Source: CAD feature listing. Evaluate the final solid. Frame: model axes, mm. A direction names the side the tool comes from. Give positions to 0.01 mm unless a question says otherwise; leave off trailing zeros. Loops run counter-clockwise (first coordinate to the right, second up) from the corner with the lowest first, then second, coordinate; pieces in that order, holes last. Notation, with made-up numbers: M 70.5,34 L 95.5,34 A28 ccw 95.5,54 Z; hole C 26.5,57 d6. An arc over 180 degrees is marked long. Answer in a Markdown table with one row per item.
```python
from build123d import *

# Parameters (mm, degrees)
ESQUISSE1_W                  = 9
ESQUISSE1_H                  = 31
BOSS_EXTRU_1_DEPTH           = 20
ESQUISSE3_W                  = 12
ESQUISSE3_H                  = 2
BOSS_EXTRU_2_DEPTH           = 15
ESQUISSE4_W                  = 12
ESQUISSE4_H                  = 2
BOSS_EXTRU_3_DEPTH           = 29.2
ESQUISSE5_R                  = 2.5
ENL_V_MAT_EXTRU_3_DEPTH      = 10
CONG_1_R                     = 2.5
CONG_2_R                     = 2.5
ENL_V_MAT_EXTRU_5_DEPTH      = 43.629642176
ENL_V_MAT_EXTRU_5_DEPTH_BACK = 5
ESQUISSE6_W                  = 7
ESQUISSE6_H                  = 11
ENL_V_MAT_EXTRU_2_DEPTH      = 43.629642176
ENL_V_MAT_EXTRU_2_DEPTH_BACK = 5
ESQUISSE2_W                  = 7
ESQUISSE2_H                  = 9


with BuildPart() as part:
    # Esquisse1 → Boss.-Extru.1 (new body)
    with BuildSketch(Plane.XY):
        Polygon((-22.275714661, 15.721830986), (-22.275714661, -12.778169014), (-22.275714661, -16.778169014), (-10.275714661, -16.778169014), (-10.275714661, 17.221830986), (-22.275714661, 17.221830986), align=None)
        with Locations((-16.275714661, 0.221830986)):
            Rectangle(ESQUISSE1_W, ESQUISSE1_H, mode=Mode.SUBTRACT)
    extrude(amount=BOSS_EXTRU_1_DEPTH)

    # Esquisse3 → Boss.-Extru.2 (add)
    with BuildSketch(Plane(origin=(0, 17.221830986, 0), x_dir=(1, 0, 0), z_dir=(0, 1, 0))):
        with Locations((-16.275714661, -5)):
            Rectangle(ESQUISSE3_W, ESQUISSE3_H)
    extrude(amount=BOSS_EXTRU_2_DEPTH)

    # Esquisse4 → Boss.-Extru.3 (add)
    with BuildSketch(Plane(origin=(0, 0, 4), x_dir=(-1, 0, 0), z_dir=(0, 0, -1))):
        with Locations((16.275714661, 31.221830986)):
            Rectangle(ESQUISSE4_W, ESQUISSE4_H)
    extrude(amount=BOSS_EXTRU_3_DEPTH)

    # Esquisse5 → Enlèv. mat.-Extru.3 (cut)
    with BuildSketch(Plane(origin=(0, 32.221830986, 0), x_dir=(1, 0, 0), z_dir=(0, 1, 0))):
        with Locations(Location((-16.275714661, 18.2, 0), (0, 0, 270))):
            Circle(ESQUISSE5_R)
    extrude(amount=-ENL_V_MAT_EXTRU_3_DEPTH, mode=Mode.SUBTRACT)

    # Congé1
    cong_1_edges = [part.edges().sort_by_distance(p)[0] for p in [
        (-10.275714661, 17.221830986, 13),
        (-10.275714661, -16.778169014, 10),
    ]]
    fillet(cong_1_edges, radius=CONG_1_R)

    # Congé2
    cong_2_edges = [part.edges().sort_by_distance(p)[0] for p in [
        (-22.275714661, 17.221830986, 13),
        (-22.275714661, -16.778169014, 10),
        (-22.275714661, 17.221830986, 2),
        (-10.275714661, 17.221830986, 2),
    ]]
    fillet(cong_2_edges, radius=CONG_2_R)

    # Esquisse6 → Enlèv. mat.-Extru.5 (cut, two sides: drawn at the far end of the back side and taken through both)
    with BuildSketch(Plane.ZY.offset(22.275714661).offset(-ENL_V_MAT_EXTRU_5_DEPTH_BACK)):
        with Locations((3.5, 1.721830986)):
            Rectangle(ESQUISSE6_W, ESQUISSE6_H)
    extrude(amount=ENL_V_MAT_EXTRU_5_DEPTH + ENL_V_MAT_EXTRU_5_DEPTH_BACK, mode=Mode.SUBTRACT)

    # Esquisse2 → Enlèv. mat.-Extru.2 (cut, two sides: drawn at the far end of the back side and taken through both)
    with BuildSketch(Plane(origin=(-10.275714661, 0, 0), x_dir=(0, 0, -1), z_dir=(1, 0, 0)).offset(-ENL_V_MAT_EXTRU_2_DEPTH_BACK)):
        with Locations((-3.5, 0.721830986)):
            Rectangle(ESQUISSE2_W, ESQUISSE2_H)
    extrude(amount=ENL_V_MAT_EXTRU_2_DEPTH + ENL_V_MAT_EXTRU_2_DEPTH_BACK, mode=Mode.SUBTRACT)


solid = part.part
```
Q1. Section query B-B (z = 2.5). Output: boundary loops of the cut face in (x, y).
Values follow:
| item | result |
|---|---|
| outline | M -22.28,-14.28 A2.5 ccw -19.78,-16.78 L -12.78,-16.78 A2.5 ccw -10.28,-14.28 L -10.28,-3.78 L -11.78,-3.78 L -11.78,-15.28 L -20.78,-15.28 L -20.78,-3.78 L -22.28,-3.78 Z; M -22.28,7.22 L -20.78,7.22 L -20.78,15.72 L -11.78,15.72 L -11.78,5.22 L -10.28,5.22 L -10.28,14.72 A2.5 ccw -12.78,17.22 L -19.78,17.22 A2.5 ccw -22.28,14.72 Z; M -22.28,30.22 L -10.28,30.22 L -10.28,32.22 L -22.28,32.22 Z |
Q2. Mould query, pull axis Y, two halves, no side actions, for faces 4 (the cylindrical face through (-10.99, 16.47, 2.03)), 5 (the cylindrical face through (-10.99, -16.03, 10.14)), 6 (the flat face through (-22, 2, 7)), 7 (the flat face through (-16, 16, 0)). Classes: +Y half, -Y half, draft (parallel to the pull), parting line (faces both ways), or undercut.
Values follow:
| item | result |
|---|---|
| face 4 | undercut |
| face 5 | -Y half |
| face 6 | undercut |
| face 7 | draft |
Q3. Section query A-A (z = -18.2). Output: boundary loops of the cut face in (x, y).
Values follow:
| item | result |
|---|---|
| outline | M -22.28,30.22 L -18.78,30.22 L -18.78,32.22 L -22.28,32.22 Z; M -13.78,30.22 L -10.28,30.22 L -10.28,32.22 L -13.78,32.22 Z |
Q4. Contact query for flat-ended pins moving along their axis: pin 1 Ø5 at (x, y) = (-15.5, -9) entering from -Z; pin 2 Ø5 at (x, y) = (-18.5, 13.5) entering from -Z; pin 3 Ø2 at (x, z) = (-14, -12.5) entering from -Y; pin 4 Ø2 at (x, z) = (-16, 10) entering from +Y. Output: stop coordinate, or through.
Values follow:
| item | result |
|---|---|
| pin 1 | through |
| pin 2 | z = 0 |
| pin 3 | y = 30.22 |
| pin 4 | y = 17.22 |
Q5. Reachability of faces 1 (the flat face through (-16, -15.278, 10)), 2 (the cylindrical face through (-10.99, 16.47, 13.1)), 3 (the flat face through (-16, 17.222, 13)) from +Z, -Z, +X, -X, +Y, -Y: full face, straight path, thin tool, end or side. Return the list, or none.
Values follow:
| item | result |
|---|---|
| face 1 | +Z, -Z |
| face 2 | +Z, +X, +Y |
| face 3 | +Z, +X, -X, +Y |
Q6. Ray query, probe 1 along Y at (x, z) = (-14, 2); probe 2 along Y at (x, z) = (-14.75, 7); probe 3 along X at (y, z) = (30.85, -18.2). Return the intervals inside material, ascending. Write a range as from..to.
Values follow:
| item | result |
|---|---|
| probe 1 | -16.78..-15.28, 15.72..17.22, 30.22..32.22 |
| probe 2 | -16.78..-15.28, 15.72..17.22 |
| probe 3 | -22.28..-18.78, -13.78..-10.28 |
Q7. Section query C-C (x = -18). Output: boundary loops of the cut face in (y, z).
Values follow:
| item | result |
|---|---|
| outline | M -16.78,0 L -15.28,0 L -15.28,20 L -16.78,20 Z; M 15.72,0 L 17.22,0 L 17.22,4 L 30.22,4 L 30.22,-16.39 L 32.22,-16.39 L 32.22,6 L 17.22,6 L 17.22,20 L 15.72,20 Z; M 30.22,-25.2 L 32.22,-25.2 L 32.22,-20.01 L 30.22,-20.01 Z |
Q8. Section query D-D (z = 17.5). Output: boundary loops of the cut face in (x, y), plus the area to 3 significant figures.
Values follow:
| item | result |
|---|---|
| outline | M -22.28,-14.28 A2.5 ccw -19.78,-16.78 L -12.78,-16.78 A2.5 ccw -10.28,-14.28 L -10.28,14.72 A2.5 ccw -12.78,17.22 L -19.78,17.22 A2.5 ccw -22.28,14.72 Z; hole M -20.78,-15.28 L -11.78,-15.28 L -11.78,15.72 L -20.78,15.72 Z |
| area | 124 mm^2 |
